```python
from build123d import *

# Parameters (mm, degrees)
F0_W     = 120.65
F0_H     = 67.31
F1_DEPTH = 6.35
F2_T     = -3.175
F3_W     = 64.135
F3_H     = 2.54
F4_DEPTH = 2.54
F4_TAPER = 20
F6_R     = 2.286
F7_DEPTH = 25.4


with BuildPart() as f1:
    # F0 (on Top) → F1 (new body, symmetric)
    with BuildSketch(Plane.XY):
        Rectangle(F0_W, F0_H)
    extrude(amount=F1_DEPTH, both=True)

    # F2
    f2_openings = [f1.faces().sort_by_distance(p)[0] for p in [
        (0, 0, 6.35),
        (0, 33.655, 0),
    ]]
    offset(amount=F2_T, openings=f2_openings)

    # F3 (on face) → F4 (join)
    with BuildSketch(Plane.YZ.offset(-57.15)):
        with Locations((1.5875, 5.08)):
            Rectangle(F3_W, F3_H)
    extrude(amount=F4_DEPTH, taper=F4_TAPER)

    # F5: F1 across plane


with BuildPart() as f1_1:
    add(f1.part)
    add(f1.part.mirror(Plane.YZ))

    # F6 (on face) → F7 (cut)
    with BuildSketch(Plane.XY.offset(-3.175)):
        with Locations((-6.35, -3.1835122595)):
            Circle(F6_R)
        with Locations((6.35, -3.1835122595)):
            Circle(F6_R)
    extrude(amount=-F7_DEPTH, mode=Mode.SUBTRACT)


solid = f1_1.part
```
Could you check a few things on this model? Use its own coordinates, in mm. A direction names the side the tool comes from. Coordinates: 2 decimals unless noted, no trailing zeros. Write each loop counter-clockwise with the first axis right and the second up, starting at its lowest first coordinate (ties: lowest second). Pieces come first, ordered by that corner, then holes. Notation, with made-up numbers: (-24.5, 33.25) - (-0.5, 33.25) arc R13 ccw to (-0.5, 45.25) - close; hole circle Ø2 at (-4.5, -8.75). An arc over 180 degrees is marked (long way). Use a Markdown table: item, result.
Q1. I'm going to push flat-ended pins straight in: pin 1 Ø4 at (x, y) = (-17, -15.5) entering from +Z (3 decimals); pin 2 Ø7.5 at (x, z) = (-8.5, 1.5) entering from +Y. Where does each tip first touch, or does it pass through?
Geometry check:
| item | result |
|---|---|
| pin 1 | stops at z = -3.175 |
| pin 2 | stops at y = -30.48 |
Q2. Thinking about a two-plate mould opening in X: for faces 1 (the flat face through (-60.325, 0, 0)), 2 (the flat face through (-1, 0, -6.35)), 3 (the flat face through (-1, 2, -3.175)), 4 (the cylindrical face through (-8.634, -3.083, -4.74)), which applies, +X half, -X half, draft (parallel to the pull), parting line (faces both ways), or undercut?
Geometry check:
| item | result |
|---|---|
| face 1 | -X half |
| face 2 | draft |
| face 3 | undercut |
| face 4 | undercut |
Q3. Imagine slicing it at B-B (x = -39). List the corners of the cut face in (y, z) for me (3 decimals).
Geometry check:
| item | result |
|---|---|
| outline | (-33.655, -6.35) - (33.655, -6.35) - (33.655, -3.175) - (-30.48, -3.175) - (-30.48, 6.35) - (-33.655, 6.35) - close |
Q4. Which directions (+Z, -Z, +X, -X, +Y, -Y) give clear straight access to the entire face, cutting with the end or side of a thin tool? Please do faces 5 (the flat face through (-57.15, 1, 0)), 6 (the flat face through (0, -32, 6.35)).
Geometry check:
| item | result |
|---|---|
| face 5 | +Y |
| face 6 | +Z, +X, -X, +Y, -Y |
Q5. Imagine slicing it at A-A (x = -6.35). List the corners of the cut face in (y, z) for me (3 decimals), and give its area (3 significant figures).
Geometry check:
| item | result |
|---|---|
| outline | (-33.655, -6.35) - (-5.47, -6.35) - (-5.47, -3.175) - (-30.48, -3.175) - (-30.48, 6.35) - (-33.655, 6.35) - close; (-0.898, -6.35) - (33.655, -6.35) - (33.655, -3.175) - (-0.898, -3.175) - close |
| area | 229 mm2 |
Q6. Please list where these lines run through material, in increasing order: L1, parallel to X at y = 6, z = 5.25 (3 decimals); L2, parallel to Y at x = 6.35, z = -5.6 (3 decimals); L3, parallel to X at y = 2, z = 1.5 (3 decimals).
Geometry check:
| item | result |
|---|---|
| L1 | x = -60.325 to -54.61, 54.61 to 60.325 |
| L2 | y = -33.655 to -5.47, -0.898 to 33.655 |
| L3 | x = -60.325 to -57.15, 57.15 to 60.325 |
